Verification items for the finished model (mm, model axes). A direction names the side the tool comes from. Give positions to 0.01 mm unless a question says otherwise; leave off trailing zeros. Loops run counter-clockwise (first coordinate to the right, second up) from the corner with the lowest first, then second, coordinate; pieces in that order, holes last. Notation, with made-up numbers: (82, -20.75) - (113, -20.75) arc R10 ccw to (113, -10.75) - close; hole circle Ø7 at (-21, 51.25). An arc over 180 degrees is marked (long way). Use one line per item in the form item = value.
```python
from build123d import *

# Parameters (mm, degrees)
SKETCH1_R           = 50.8
BOSS_EXTRUDE1_DEPTH = 9.525
SKETCH2_R           = 3.175
BOSS_EXTRUDE2_DEPTH = 9.525
SKETCH7_R           = 4.7625
SKETCH7_W           = 5.08
SKETCH7_H           = 10.16
CUT_EXTRUDE10_DEPTH = 9.525


with BuildPart() as part:
    # Sketch1 → Boss-Extrude1 (new body)
    with BuildSketch(Plane.XY):
        with Locations(Location((0, 0, 0), (0, 0, 180))):
            Circle(SKETCH1_R)
    extrude(amount=BOSS_EXTRUDE1_DEPTH)

    # Sketch2 → Boss-Extrude2 (add)
    with BuildSketch(Plane.XY.offset(9.525)):
        with BuildLine():
            ThreePointArc((-28.469166667, 25.320279408), (-19.197370761, 14.139745253), (-15.875, 0))
            ThreePointArc((-15.875, 0), (-19.197370761, -14.139745253), (-28.469166667, -25.320279408))
            ThreePointArc((-28.469166667, -25.320279408), (38.1, 0), (-28.469166667, 25.320279408))
        make_face()
        with Locations(Location((-47.625, 0, 0), (0, 0, 179.999530418))):
            Circle(SKETCH2_R)
    extrude(amount=BOSS_EXTRUDE2_DEPTH)

    # Sketch7 → Cut-Extrude10 (cut)
    with BuildSketch(Plane(origin=(0, 0, 0), x_dir=(-1, 0, 0), z_dir=(0, 0, -1))):
        Circle(SKETCH7_R)
        with Locations((0, 5.08)):
            Rectangle(SKETCH7_W, SKETCH7_H)
    extrude(amount=-CUT_EXTRUDE10_DEPTH, mode=Mode.SUBTRACT)


solid = part.part
```
1. Section check D-D, the plane z = 13. Record the cut outline in (x, y) (3 decimals), then the cut area to 3 significant figures.
Result set:
outline = circle Ø6.35 at (-47.625, 0); (-28.469, -25.32) arc R38.1 ccw (long way) to (-28.469, 25.32) arc R31.75 cw to start
area = 3,810 mm²
2. Depth check by flat-ended pin: pin 1 Ø6 at (x, z) = (27, 2) entering from +Y; pin 2 Ø4 at (x, z) = (-12, 2) entering from -Y; pin 3 Ø10 at (x, y) = (12, -7) entering from -Z; pin 4 Ø4 at (x, z) = (0.5, 6) entering from -Y. Enter the tip coordinate at first touch or a pass-through.
Result set:
pin_1 = 44.77
pin_2 = -49.81
pin_3 = 0
pin_4 = -50.8
3. Scan lines: probe 1 along Y at (x, z) = (0, 4); probe 2 along Z at (x, y) = (-29.5, 37.5) (3 decimals); probe 3 along X at (y, z) = (-0.5, 7). Record each from-to range of solid material in increasing order.
Result set:
probe_1 = -50.8 to -4.76, 10.16 to 50.8
probe_2 = 0 to 9.525
probe_3 = -50.8 to -4.74, 4.74 to 50.8
4. Draft check along X on faces 4 (the flat face through (4, 1, 19.05)), 5 (the flat face through (0, 10.16, 5)), 6 (the cylindrical face through (-23.44, 45.07, 4.7)). Enter one of: released by +X, released by -X, zero draft, split by the parting line, or undercut.
Result set:
face_4 = zero draft
face_5 = undercut
face_6 = split by the parting line
5. Tool access check on faces 1 (the flat face through (-22, -1, 9.525)), 2 (the flat face through (-48, 0, 19.05)), 3 (the cylindrical face through (0.17, -4.76, 4.7)). Record the directions out of +Z, -Z, +X, -X, +Y, -Y that give a thin tool (end or side, any length) a straight path to the whole face; none if there is none.
Result set:
face_1 = +Z
face_2 = +Z, +X, -X, +Y, -Y
face_3 = -Z
6. Section check B-B, the plane z = 4.25. Record the cut outline in (x, y) (1 decimal), then the cut area to 3 significant figures.
Result set:
outline = circle Ø101.6 at (0, 0); hole (-2.5, 4) arc R4.8 ccw (long way) to (2.5, 4) - (2.5, 10.2) - (-2.5, 10.2) - close
area = 8,010 mm²
7. Section check C-C, the plane y = -33. Record the cut outline in (x, z) (3 decimals).
Result set:
outline = (-38.622, 0) - (38.622, 0) - (38.622, 9.525) - (19.042, 9.525) - (19.042, 19.05) - (-19.042, 19.05) - (-19.042, 9.525) - (-38.622, 9.525) - close
